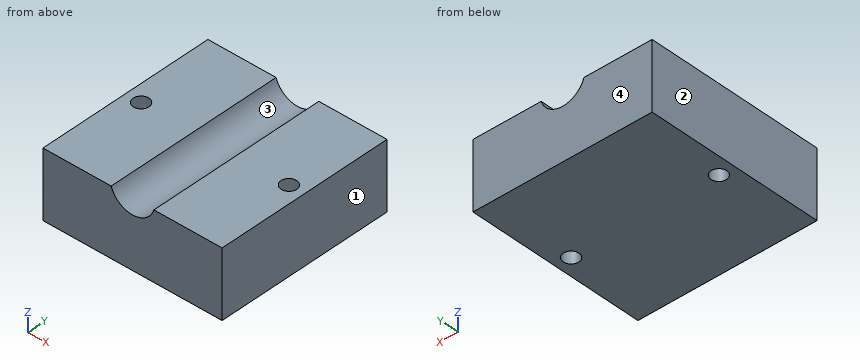
from build123d import *

# Parameters (mm, degrees)
SKETCH1_W           = 40
SKETCH1_H           = 40
BOSS_EXTRUDE1_DEPTH = 15
SKETCH2_R           = 1.75
CUT_EXTRUDE1_DEPTH  = 16
SKETCH3_R           = 5
CUT_EXTRUDE2_DEPTH  = 41


with BuildPart() as part:
    # Sketch1 → Boss-Extrude1 (new body)
    with BuildSketch(Plane.XY):
        Rectangle(SKETCH1_W, SKETCH1_H)
    extrude(amount=BOSS_EXTRUDE1_DEPTH)

    # Sketch2 → Cut-Extrude1 (cut, through all)
    with BuildSketch(Plane.XY.offset(15)):
        with Locations((-16.5, 0)):
            Circle(SKETCH2_R)
        with Locations((16.5, 0)):
            Circle(SKETCH2_R)
    extrude(amount=-CUT_EXTRUDE1_DEPTH, mode=Mode.SUBTRACT)

    # Sketch3 → Cut-Extrude2 (cut, through all)
    with BuildSketch(Plane(origin=(0, 20, 0), x_dir=(1, 0, 0), z_dir=(0, 1, 0))):
        with Locations((0, -16.5)):
            Circle(SKETCH3_R)
    extrude(amount=-CUT_EXTRUDE2_DEPTH, mode=Mode.SUBTRACT)


solid = part.part
CAD build for the part. Positions are in the model's coordinates, mm. Face numbers are marked on the shaded views. Round coordinates to 2 decimals unless told otherwise and drop trailing zeros. Order: outer loops, then holes, each group sorted by start corner. A loop starts at its lowest first (then second) coordinate and runs counter-clockwise, first axis right, second up. Notation, with made-up numbers: (78, -5.5) -> (134, -5.5) arc R23 ccw to (134, 28.5) -> close; hole circle Ø11 at (-26, 52.25). An arc over 180 degrees is marked (long way). Write item = value, one per line. Start each with the question number.
(1) Cut at A-A, the plane z = 13.5. List the corners of the cut face in (x, y), then the cut area to 3 significant figures.
(2) Pin check, flat tip, straight feed: P1, Ø5, axis at x = -3, y = -9, coming from the +Z side. Stop position of the tip, or through.
(3) Cut at C-C, the plane y = 0. List the corners of the cut face in (x, z).
(4) Pull direction X, two halves, no side cores. Call the marked faces 1, 2, 3 and 4: released by +X, released by -X, zero draft, split by the parting line, or undercut.
(5) Probe line 1 (Y direction, x = 16.5, z = 5); line 2 (Z direction, x = 2.5, y = -14); line 3 (Z direction, x = -1.5, y = -15). List the from-to ranges inside material, lowest first. Write a range as [from, to].
(6) Cut at D-D, the plane y = -13.5. List the corners of the cut face in (x, z), then the cut area to 3 significant figures.
(7) Cut at B-B, the plane x = -16.5. List the corners of the cut face in (y, z).
Model answer:
q1.outline = (-20, -20) -> (-4, -20) -> (-4, 20) -> (-20, 20) -> close; (4, -20) -> (20, -20) -> (20, 20) -> (4, 20) -> close; hole circle Ø3.5 at (-16.5, 0); hole circle Ø3.5 at (16.5, 0)
q1.area = 1,260 mm2
q2.P1 = 15
q3.outline = (-20, 0) -> (-18.25, 0) -> (-18.25, 15) -> (-20, 15) -> close; (-14.75, 0) -> (14.75, 0) -> (14.75, 15) -> (4.77, 15) arc R5 cw to (-4.77, 15) -> (-14.75, 15) -> close; (18.25, 0) -> (20, 0) -> (20, 15) -> (18.25, 15) -> close
q4.face_1 = released by +X
q4.face_2 = released by -X
q4.face_3 = undercut
q4.face_4 = zero draft
q5.line_1 = [-20, -1.75], [1.75, 20]
q5.line_2 = [0, 12.17]
q5.line_3 = [0, 11.73]
q6.outline = (-20, 0) -> (20, 0) -> (20, 15) -> (4.77, 15) arc R5 cw to (-4.77, 15) -> (-20, 15) -> close
q6.area = 576 mm2
q7.outline = (-20, 0) -> (-1.75, 0) -> (-1.75, 15) -> (-20, 15) -> close; (1.75, 0) -> (20, 0) -> (20, 15) -> (1.75, 15) -> close
